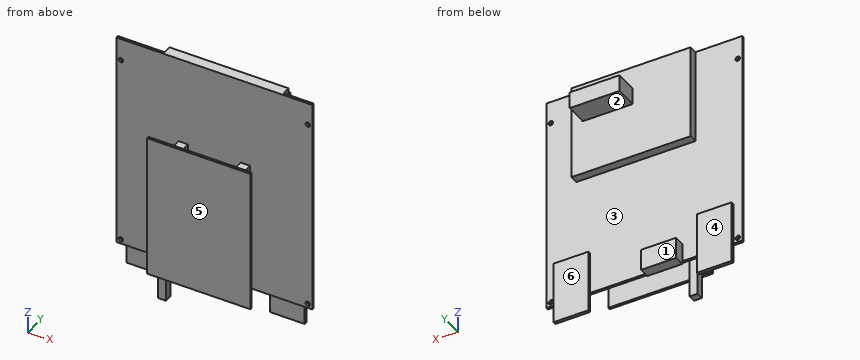
from build123d import *

# Parameters (mm, degrees)
ESQUISSE1_W        = 130
ESQUISSE1_H        = 145
ESQUISSE1_R        = 1.5
BOSS_EXTRU_1_DEPTH = 1.6
ESQUISSE2_W        = 79
ESQUISSE2_H        = 63
BOSS_EXTRU_2_DEPTH = 5.5
ESQUISSE3_W        = 33.047140846
ESQUISSE3_H        = 11.107836296
BOSS_EXTRU_3_DEPTH = 14.8
ESQUISSE4_W        = 23.239665889
ESQUISSE4_H        = 14.216628141
BOSS_EXTRU_4_DEPTH = 7
ESQUISSE5_W        = 23
ESQUISSE5_H        = 41.525911652
BOSS_EXTRU_5_DEPTH = 2
ESQUISSE6_W        = 6.210910455
ESQUISSE6_H        = 46.190495577
BOSS_EXTRU_6_DEPTH = 17.7
ESQUISSE7_W        = 68.5
ESQUISSE7_H        = 96
BOSS_EXTRU_7_DEPTH = 1.6
ESQUISSE8_W        = 5.226174608
ESQUISSE8_H        = 26.34937469
BOSS_EXTRU_8_DEPTH = 5


with BuildPart() as part:
    # Esquisse1 → Boss.-Extru.1 (new body)
    with BuildSketch(Plane(origin=(0, 0, 0), x_dir=(1, 0, 0), z_dir=(0, 1, 0))):
        with Locations((0, 72.5)):
            Rectangle(ESQUISSE1_W, ESQUISSE1_H)
        with Locations((-62, 142)):
            Circle(ESQUISSE1_R, mode=Mode.SUBTRACT)
        with Locations((62, 142)):
            Circle(ESQUISSE1_R, mode=Mode.SUBTRACT)
        with Locations((62, 15)):
            Circle(ESQUISSE1_R, mode=Mode.SUBTRACT)
        with Locations((-62, 15)):
            Circle(ESQUISSE1_R, mode=Mode.SUBTRACT)
    extrude(amount=BOSS_EXTRU_1_DEPTH)

    # Esquisse2 → Boss.-Extru.2 (add)
    with BuildSketch(Plane(origin=(0, 1.6, 0), x_dir=(1, 0, 0), z_dir=(0, 1, 0))):
        with Locations((5.5, 31.5)):
            Rectangle(ESQUISSE2_W, ESQUISSE2_H)
    extrude(amount=BOSS_EXTRU_2_DEPTH)

    # Esquisse3 → Boss.-Extru.3 (add)
    with BuildSketch(Plane(origin=(0, 7.1, 0), x_dir=(1, 0, 0), z_dir=(0, 1, 0))):
        with Locations((21.089415125, 20.538253018)):
            Rectangle(ESQUISSE3_W, ESQUISSE3_H)
    extrude(amount=BOSS_EXTRU_3_DEPTH)

    # Esquisse4 → Boss.-Extru.4 (add)
    with BuildSketch(Plane(origin=(0, 1.6, 0), x_dir=(1, 0, 0), z_dir=(0, 1, 0))):
        with Locations((-13.559579353, 139.891685929)):
            Rectangle(ESQUISSE4_W, ESQUISSE4_H)
    extrude(amount=BOSS_EXTRU_4_DEPTH)

    # Esquisse5 → Boss.-Extru.5 (add)
    with BuildSketch(Plane(origin=(0, 1.6, 0), x_dir=(1, 0, 0), z_dir=(0, 1, 0))):
        with Locations((-47.5, 137.737044174)):
            Rectangle(ESQUISSE5_W, ESQUISSE5_H)
        with Locations((47.5, 137.737044174)):
            Rectangle(ESQUISSE5_W, ESQUISSE5_H)
    extrude(amount=BOSS_EXTRU_5_DEPTH)

    # Esquisse6 → Boss.-Extru.6 (add)
    with BuildSketch(Plane.XZ):
        with Locations((20.563763626, -81.400742682)):
            Rectangle(ESQUISSE6_W, ESQUISSE6_H)
        with Locations((-20.563763626, -81.400742682)):
            Rectangle(ESQUISSE6_W, ESQUISSE6_H)
    extrude(amount=BOSS_EXTRU_6_DEPTH)

    # Esquisse7 → Boss.-Extru.7 (add)
    with BuildSketch(Plane.XZ.offset(17.7)):
        with Locations((0, -97)):
            Rectangle(ESQUISSE7_W, ESQUISSE7_H)
    extrude(amount=-BOSS_EXTRU_7_DEPTH)

    # Esquisse8 → Boss.-Extru.8 (add)
    with BuildSketch(Plane(origin=(0, -16.1, 0), x_dir=(1, 0, 0), z_dir=(0, 1, 0))):
        with Locations((-25.296871339, 147.825312655)):
            Rectangle(ESQUISSE8_W, ESQUISSE8_H)
    extrude(amount=BOSS_EXTRU_8_DEPTH)


solid = part.part
The model under review builds one solid part; all positions refer to its coordinate system, in mm. Face numbers are marked on the shaded views. A direction names the side the tool comes from. Give positions to 0.01 mm unless a question says otherwise; leave off trailing zeros. Order: outer loops, then holes, each group sorted by start corner. A loop starts at its lowest first (then second) coordinate and runs counter-clockwise, first axis right, second up. Notation, with made-up numbers: (65, 20) -> (85, 20) arc R19 cw to (85, 49) -> close; hole circle Ø8 at (36, -14.75). An arc over 180 degrees is marked (long way). Write item = value, one per line. Start each with the question number.
(1) For L1, parallel to Z at x = 62, y = 1.05; L2, parallel to X at y = 0.4, z = -142; L3, parallel to Y at x = 10, z = -88, list the stretches that pass through material, from the lowest coordinate up. Write a range as from..to.
(2) Tool access review of the marked faces 4, 5 and 6: name each direction out of +Z, -Z, +X, -X, +Y, -Y from which nothing blocks a thin tool from reaching the whole face with its end or side.
(3) Draft analysis for pull direction Z (two halves, no side actions). For the marked faces 1, 2 and 3, state which applies: +Z half, -Z half, draft (parallel to the pull), parting line (faces both ways), or undercut.
(4) Take a section at C-C (x = 40). Write out the cut boundary in (y, z).
(5) For pin 1 Ø5 at (x, y) = (-41.5, 4.5) entering from -Z; pin 2 Ø3 at (x, z) = (-47.5, -113) entering from +Y; pin 3 Ø15.5 at (x, z) = (-13, -138.5) entering from +Y; pin 4 Ø10 at (x, y) = (-35.5, 16.5) entering from -Z, all flat-tipped, find the tip position at first contact; note any pin that passes through.
(6) Take a section at B-B (x = -15.5). Write out the cut boundary in (y, z), plus the area to 3 significant figures.
(7) Take a section at A-A (z = -84). Write out the cut boundary in (x, y).
Returned:
q1.L1 = -145..-143.5, -140.5..-16.5, -13.5..0
q1.L2 = -65..-63.5, -60.5..60.5, 63.5..65
q1.L3 = -17.7..-16.1, 0..1.6
q2.face_4 = +Z, -Z, -X, +Y
q2.face_5 = +Z, -Z, +X, -X, -Y
q2.face_6 = -Z, +X, +Y
q3.face_1 = draft
q3.face_2 = -Z half
q3.face_3 = undercut
q4.outline = (0, -145) -> (1.6, -145) -> (1.6, -158.5) -> (3.6, -158.5) -> (3.6, -116.97) -> (1.6, -116.97) -> (1.6, -63) -> (7.1, -63) -> (7.1, 0) -> (0, 0) -> close
q5.pin_1 = -158.5
q5.pin_2 = 1.6
q5.pin_3 = 8.6
q5.pin_4 = through
q6.outline = (-17.7, -145) -> (-16.1, -145) -> (-16.1, -49) -> (-17.7, -49) -> close; (0, -145) -> (1.6, -145) -> (1.6, -147) -> (8.6, -147) -> (8.6, -132.78) -> (1.6, -132.78) -> (1.6, -63) -> (7.1, -63) -> (7.1, 0) -> (0, 0) -> close
q6.area = 832 mm²
q7.outline = (-65, 0) -> (-23.67, 0) -> (-23.67, -16.1) -> (-34.25, -16.1) -> (-34.25, -17.7) -> (34.25, -17.7) -> (34.25, -16.1) -> (23.67, -16.1) -> (23.67, 0) -> (65, 0) -> (65, 1.6) -> (-65, 1.6) -> close; hole (-17.46, -16.1) -> (17.46, -16.1) -> (17.46, 0) -> (-17.46, 0) -> close
